Geometry check sheet. Reference: drawing and pictorial views, mm from the part's lowest x, y, z. Give positions to 0.01 mm unless a question says otherwise; leave off trailing zeros. Order: outer loops, then holes, each group sorted by start corner. A loop starts at its lowest first (then second) coordinate and runs counter-clockwise, first axis right, second up. Notation, with made-up numbers: M 12.25,-19.5 L 35.25,-19.5 A16 ccw 35.25,9.5 Z; hole C -36,-13 d2. An arc over 180 degrees is marked long. Answer as CSV lines item,"result".
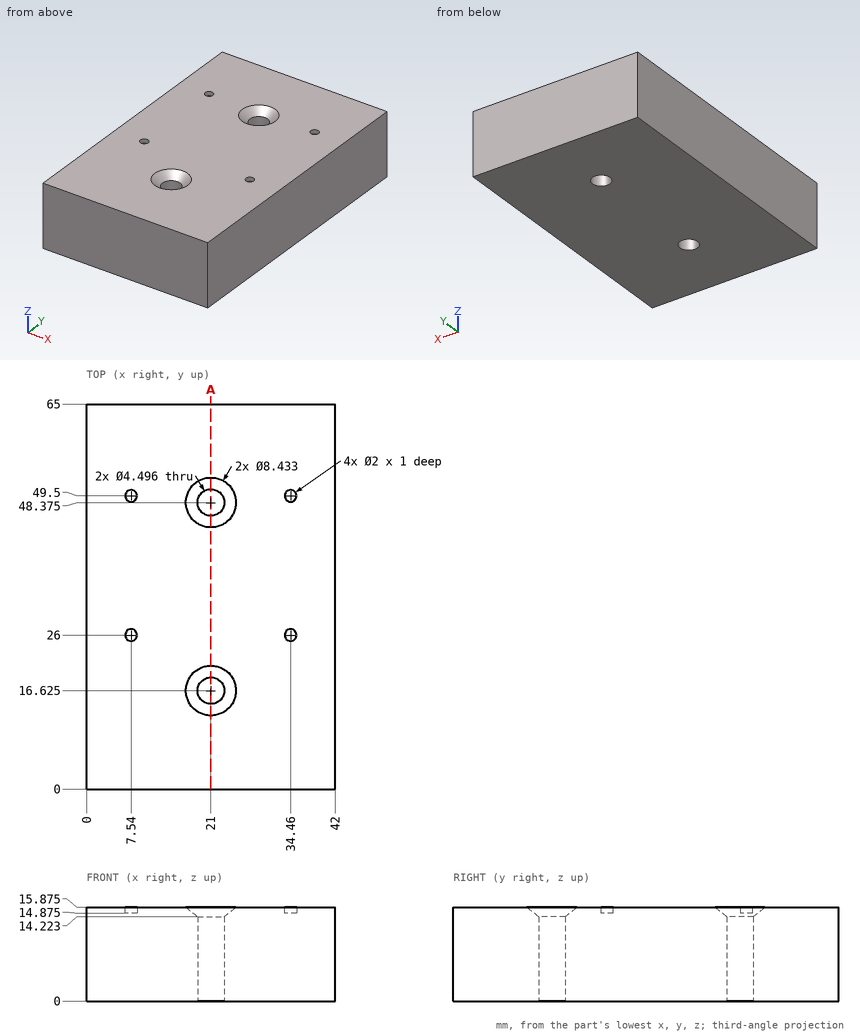
(1) Gauge pin test, flat ends, axial feed: P1, Ø3, axis at x = 34.46, y = 49.5, coming from the +Z side (3 decimals); P2, Ø1.2, axis at x = 7.54, y = 49.5, coming from the +Z side (3 decimals). Record the tip position at first contact, or that the pin passes through.
The answers:
P1,"stops at z = 15.875"
P2,"stops at z = 14.875"
(2) Section check A-A on x = 21. Enter the section's corners in (y, z) (1 decimal).
The answers:
outline,"M 0,0 L 14.4,0 L 14.4,14.2 L 12.4,15.9 L 0,15.9 Z; M 18.9,0 L 46.1,0 L 46.1,14.2 L 44.2,15.9 L 20.8,15.9 L 18.9,14.2 Z; M 50.6,0 L 65,0 L 65,15.9 L 52.6,15.9 L 50.6,14.2 Z"
(3) Material ranges on line 1 (Y direction, x = 21, z = 9); line 2 (Y direction, x = 20.5, z = 11.5); line 3 (X direction, y = 18.5, z = 10.25), recorded low to high.
The answers:
line 1,"y = 0 to 14.38, 18.87 to 46.13, 50.62 to 65"
line 2,"y = 0 to 14.43, 18.82 to 46.18, 50.57 to 65"
line 3,"x = 0 to 19.76, 22.24 to 42"
